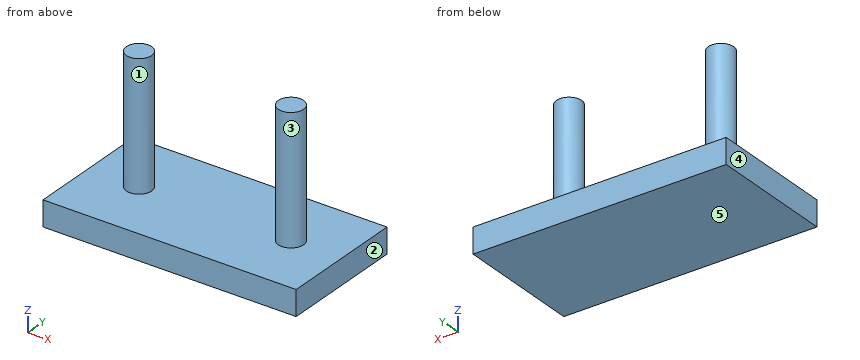
```python
from build123d import *

# Parameters (mm, degrees)
SKETCH1_W           = 100
SKETCH1_H           = 50
SKETCH1_R           = 5
BOSS_EXTRUDE1_DEPTH = 10
SKETCH1_3_R         = 5
BOSS_EXTRUDE2_DEPTH = 60


with BuildPart() as part:
    # Sketch1 → Boss-Extrude1 (new body)
    # profile 1 of 3: a face of its own
    with BuildSketch(Plane.XY):
        Rectangle(SKETCH1_W, SKETCH1_H)
        with Locations((30, 0)):
            Circle(SKETCH1_R, mode=Mode.SUBTRACT)
        with Locations((-30, 0)):
            Circle(SKETCH1_R, mode=Mode.SUBTRACT)
    # profile 2 of 3: a face of its own
    with BuildSketch(Plane.XY):
        with Locations((30, 0)):
            Circle(SKETCH1_R)
    # profile 3 of 3: a face of its own
    with BuildSketch(Plane.XY):
        with Locations((-30, 0)):
            Circle(SKETCH1_R)
    extrude(amount=BOSS_EXTRUDE1_DEPTH)

    # Sketch1_3 → Boss-Extrude2 (add)
    with BuildSketch(Plane.XY):
        with Locations((-30, 0)):
            Circle(SKETCH1_3_R)
        with Locations((30, 0)):
            Circle(SKETCH1_3_R)
    extrude(amount=BOSS_EXTRUDE2_DEPTH)


solid = part.part
```
Geometry: final body of the model. Coordinates: model frame, mm. Face numbers are marked on the shaded views. A direction names the side the tool comes from. Give positions to 0.01 mm unless a question says otherwise; leave off trailing zeros. Loops run counter-clockwise (first coordinate to the right, second up) from the corner with the lowest first, then second, coordinate; pieces in that order, holes last. Notation, with made-up numbers: (18, -31) - (50, -31) arc R19 ccw to (50, -10) - close; hole circle Ø2 at (36, 34). An arc over 180 degrees is marked (long way). Answer as CSV lines item,"result". Start each with the question number.
(1) Reachability of the marked faces 1 and 2 from +Z, -Z, +X, -X, +Y, -Y: full face, straight path, thin tool, end or side. Return the list, or none.
(2) Mould query, pull axis X, two halves, no side actions, for the marked faces 3, 4 and 5. Classes: +X half, -X half, draft (parallel to the pull), parting line (faces both ways), or undercut.
(3) Section query A-A (x = -30). Output: boundary loops of the cut face in (y, z), and give its area (3 significant figures).
(4) Section query C-C (z = 45). Output: boundary loops of the cut face in (x, y).
(5) Section query B-B (y = 0). Output: boundary loops of the cut face in (x, z).
(6) Section query D-D (x = -15). Output: boundary loops of the cut face in (y, z), and give its area (3 significant figures).
(7) Pin query (flat end, axial travel): P1, Ø8, axis at x = 4.5, y = 11.5, coming from the +Z side; P2, Ø6, axis at x = 36.5, y = -3, coming from the -Z side; P3, Ø3, axis at x = -30.5, z = 14, coming from the +Y side. Return the tip coordinate at first contact, or that it passes through.
(8) Ray query, line 1 along Z through (x, y) = (-8, -14.5); line 2 along X through (y, z) = (1, 20.5); line 3 along Y through (x, z) = (-32, 56.5). Return the intervals inside material, ascending. Write a range as [from, to].
Worked answers:
1,face 1,"+Z"
1,face 2,"+Z, -Z, +X, +Y, -Y"
2,face 3,"undercut"
2,face 4,"-X half"
2,face 5,"draft"
3,outline,"(-25, 0) - (25, 0) - (25, 10) - (5, 10) - (5, 60) - (-5, 60) - (-5, 10) - (-25, 10) - close"
3,area,"1,000 mm^2"
4,outline,"circle Ø10 at (-30, 0); circle Ø10 at (30, 0)"
5,outline,"(-50, 0) - (50, 0) - (50, 10) - (35, 10) - (35, 60) - (25, 60) - (25, 10) - (-25, 10) - (-25, 60) - (-35, 60) - (-35, 10) - (-50, 10) - close"
6,outline,"(-25, 0) - (25, 0) - (25, 10) - (-25, 10) - close"
6,area,"500 mm^2"
7,P1,"stops at z = 10"
7,P2,"stops at z = 0"
7,P3,"stops at y = 5"
8,line 1,"z = [0, 10]"
8,line 2,"x = [-34.9, -25.1], [25.1, 34.9]"
8,line 3,"y = [-4.58, 4.58]"
